from build123d import *

# Parameters (mm, degrees)
SZKIC1_R                        = 23.5
DODANIE_WYCI_GNI_CIE1_DEPTH     = 302
SZKIC2_R                        = 17.5
DODANIE_WYCI_GNI_CIE2_DEPTH     = 50
SZKIC4_R                        = 17.5
DODANIE_WYCI_GNI_CIE3_DEPTH     = 50
SZKIC5_R                        = 5.05
WYTNIJ_WYCI_GNI_CIE1_DEPTH      = 50
SFAZOWANIE1_SIZE                = 2
SZKIC8_R                        = 24
DODANIE_WYCI_GNI_CIE4_DEPTH     = 42.129872
SZKIC12_R                       = 7
DODANIE_WYCI_GNI_CIE5_DEPTH     = 61.69017
SZKIC6_R                        = 11
WYTNIJ_WYCI_GNI_CIE2_DEPTH      = 302
SZKIC13_R                       = 7
DODANIE_WYCI_GNI_CIE6_DEPTH     = 50
DODANIE_WYCI_GNI_CIE7_START     = 14.5
DODANIE_WYCI_GNI_CIE7_DEPTH     = 3
ZAOKR_GLENIE1_R                 = 10
LUSTRO2_START                   = 14.5
LUSTRO2_COPY_1_DEPTH            = 3
WYTNIJ_WYCI_GNI_CIE3_START      = -3
SZKIC17_R                       = 23.5
SZKIC17_R_2                     = 23
WYTNIJ_WYCI_GNI_CIE3_DEPTH      = 8
SZKIC18_R                       = 23.5
SZKIC18_R_2                     = 17
WYTNIJ_WYCI_GNI_CIE4_DEPTH      = 60
WYTNIJ_WYCI_GNI_CIE4_DEPTH_BACK = 95
SZKIC20_R                       = 18.5
WYTNIJ_WYCI_GNI_CIE5_DEPTH      = 45


with BuildPart() as part:
    # Szkic1 → Dodanie-wyciągnięcie1 (new body)
    with BuildSketch(Plane(origin=(0, 0, 0), x_dir=(0, 0, -1), z_dir=(1, 0, 0))):
        Circle(SZKIC1_R)
    extrude(amount=DODANIE_WYCI_GNI_CIE1_DEPTH)

    # Szkic2 → Dodanie-wyciągnięcie2 (add)
    with BuildSketch(Plane.XY):
        with Locations((31, -38)):
            Circle(SZKIC2_R)
    extrude(amount=DODANIE_WYCI_GNI_CIE2_DEPTH)

    # Szkic4 → Dodanie-wyciągnięcie3 (add)
    with BuildSketch(Plane(origin=(0, 0, 0), x_dir=(-1, 0, 0), z_dir=(0, 0, -1))):
        with Locations((-271, -38)):
            Circle(SZKIC4_R)
    extrude(amount=-DODANIE_WYCI_GNI_CIE3_DEPTH)

    # Szkic5 → Wytnij-wyciągnięcie1 (cut)
    with BuildSketch(Plane.XY.offset(50)):
        with Locations((31, -38)):
            Circle(SZKIC5_R)
        with Locations((271, -38)):
            Circle(SZKIC5_R)
    extrude(amount=-WYTNIJ_WYCI_GNI_CIE1_DEPTH, mode=Mode.SUBTRACT)

    # Sfazowanie1
    sfazowanie1_edges = [part.edges().sort_by_distance(p)[0] for p in [
        (25.95, -38, 0),
        (25.95, -38, 50),
        (265.95, -38, 0),
        (265.95, -38, 50),
    ]]
    chamfer(sfazowanie1_edges, length=SFAZOWANIE1_SIZE)

    # Szkic8 → Dodanie-wyciągnięcie4 (add)
    with BuildSketch(Plane(origin=(64.694528313, 23.5, 42), x_dir=(0.996917334, 0, 0.078459096), z_dir=(-0.078459096, 0, 0.996917334))):
        with Locations((0, -13.25)):
            Circle(SZKIC8_R)
    extrude(amount=-DODANIE_WYCI_GNI_CIE4_DEPTH)

    # Szkic12 → Dodanie-wyciągnięcie5 (add)
    with BuildSketch(Plane(origin=(-2.886875267, 0, 36.681228189), x_dir=(0.996917334, 0, 0.078459096), z_dir=(-0.078459096, 0, 0.996917334))):
        with Locations((67.790378694, 10.25)):
            Circle(SZKIC12_R)
    extrude(amount=DODANIE_WYCI_GNI_CIE5_DEPTH)

    # Szkic6 → Wytnij-wyciągnięcie2 (cut)
    with BuildSketch(Plane.ZY):
        Circle(SZKIC6_R)
    extrude(amount=-WYTNIJ_WYCI_GNI_CIE2_DEPTH, mode=Mode.SUBTRACT)

    # Szkic13 → Dodanie-wyciągnięcie6 (add)
    with BuildSketch(Plane(origin=(64.694528313, 23.5, 42), x_dir=(0.996917334, 0, 0.078459096), z_dir=(-0.078459096, 0, 0.996917334))):
        with Locations((0, -13.25)):
            Circle(SZKIC13_R)
    extrude(amount=-DODANIE_WYCI_GNI_CIE6_DEPTH)

    # Szkic16 → Dodanie-wyciągnięcie7 (add)
    with BuildSketch(Plane.ZY.offset(-31).offset(DODANIE_WYCI_GNI_CIE7_START)):
        Polygon((50, -38), (0, -38), (0, -20.172556468), (13.849344331, -17.060101722), (21.580694053, -1.91951259), (17.483252048, 15.703053774), (50, -20.5), align=None)
    dodanie_wyci_gni_cie7 = extrude(amount=DODANIE_WYCI_GNI_CIE7_DEPTH)

    # Zaokrąglenie1
    zaokr_glenie1_edges = [part.edges().sort_by_distance(p)[0] for p in [
        (68.000000001, 34.25, 3.37e-07),
    ]]
    fillet(zaokr_glenie1_edges, radius=ZAOKR_GLENIE1_R)

    # Lustro1: Dodanie-wyciągnięcie7 across plane
    add(dodanie_wyci_gni_cie7.mirror(Plane.ZY.offset(-31)))

    # Lustro2: Dodanie-wyciągnięcie7 across plane
    add(dodanie_wyci_gni_cie7.mirror(Plane.ZY.offset(-151)))

    # Lustro2 copy 1 sketch → Lustro2 copy 1 (add)
    with BuildSketch(Plane.ZY.offset(-271).offset(LUSTRO2_START)):
        Polygon((50, -38), (0, -38), (0, -20.172556468), (13.849344331, -17.060101722), (21.580694053, -1.91951259), (17.483252048, 15.703053774), (50, -20.5), align=None)
    extrude(amount=LUSTRO2_COPY_1_DEPTH)

    # Szkic17 → Wytnij-wyciągnięcie3 (cut)
    with BuildSketch(Plane.ZY.offset(WYTNIJ_WYCI_GNI_CIE3_START)):
        Circle(SZKIC17_R)
        Circle(SZKIC17_R_2, mode=Mode.SUBTRACT)
    wytnij_wyci_gni_cie3 = extrude(amount=-WYTNIJ_WYCI_GNI_CIE3_DEPTH, mode=Mode.SUBTRACT)

    # Lustro3: Wytnij-wyciągnięcie3 across plane
    add(wytnij_wyci_gni_cie3.mirror(Plane.ZY.offset(-151)), mode=Mode.SUBTRACT)

    # Szkic18 → Wytnij-wyciągnięcie4 (cut, two sides)
    with BuildSketch(Plane.ZY.offset(-151)) as wytnij_wyci_gni_cie4_sk:
        Circle(SZKIC18_R)
        Circle(SZKIC18_R_2, mode=Mode.SUBTRACT)
    extrude(amount=WYTNIJ_WYCI_GNI_CIE4_DEPTH, mode=Mode.SUBTRACT)
    extrude(wytnij_wyci_gni_cie4_sk.sketch, amount=-WYTNIJ_WYCI_GNI_CIE4_DEPTH_BACK, mode=Mode.SUBTRACT)

    # Szkic19 → Obrót1 (revolve)
    with BuildSketch(Plane.XY):
        Polygon((91, 23.5), (91, 17), (121, 17), align=None)
        Polygon((246, 17), (246, 23.5), (236, 17), align=None)
    revolve(axis=Axis((0, 0, 0), (1, 0, 0)))

    # Szkic20 → Wytnij-wyciągnięcie5 (cut)
    with BuildSketch(Plane.ZY):
        Circle(SZKIC20_R)
    wytnij_wyci_gni_cie5 = extrude(amount=-WYTNIJ_WYCI_GNI_CIE5_DEPTH, mode=Mode.SUBTRACT)

    # Lustro4: Wytnij-wyciągnięcie5 across plane
    add(wytnij_wyci_gni_cie5.mirror(Plane.ZY.offset(-151)), mode=Mode.SUBTRACT)


solid = part.part
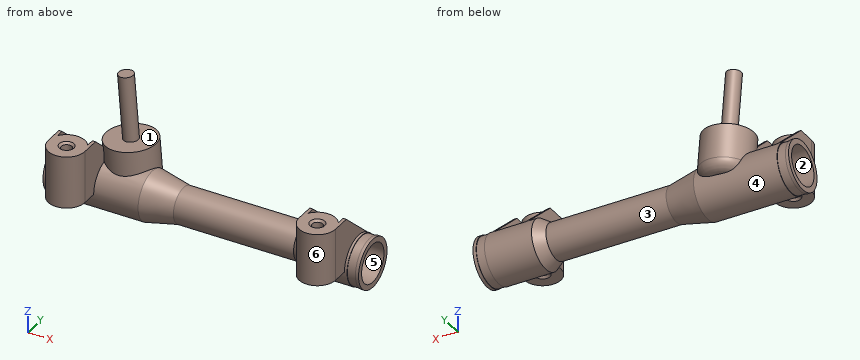
Check sheet for the modelled part. Datum: model origin and axes. Units: mm. Face numbers are marked on the shaded views. A direction names the side the tool comes from. Give positions to 0.01 mm unless a question says otherwise; leave off trailing zeros. Order: outer loops, then holes, each group sorted by start corner. A loop starts at its lowest first (then second) coordinate and runs counter-clockwise, first axis right, second up. Notation, with made-up numbers: (30.5, 45.25) - (43.5, 45.25) arc R9 ccw to (43.5, 51.25) - close; hole circle Ø5 at (47.5, -24). An arc over 180 degrees is marked (long way). Answer as CSV lines item,"result".
1. Mould release check, pull along Y, two halves, no side actions. Record for the marked faces 1, 2 and 3: released by +Y, released by -Y, zero draft, split by the parting line, or undercut.
Result sheet:
face 1,"zero draft"
face 2,"undercut"
face 3,"split by the parting line"
2. Tool access check on the marked faces 4, 5 and 6. Record the directions out of +Z, -Z, +X, -X, +Y, -Y that give a thin tool (end or side, any length) a straight path to the whole face; none if there is none.
Result sheet:
face 4,"none"
face 5,"+X"
face 6,"+Z, -Z, -Y"
3. Go/stop test with flat-tipped pins: P1, Ø5, axis at y = 8.5, z = 11, coming from the +X side; P2, Ø11.5, axis at x = 31, y = -38, coming from the -Z side; P3, Ø15, axis at y = -7, z = 34.5, coming from the +X side; P4, Ø12, axis at x = 243.5, y = -33, coming from the -Z side. Record where each tip stops, or that it passes through.
Result sheet:
P1,"x = 257"
P2,"z = 1.3"
P3,"x = 288.5"
P4,"through"
4. Section check A-A (x = 31). Record the boundary of the cut face in (y, z).
Result sheet:
outline,"(-55.5, 0) - (-45.05, 0) - (-43.05, 2) - (-43.05, 48) - (-45.05, 50) - (-55.5, 50) - close; (-32.95, 2) - (-30.95, 0) - (-23.5, 0) arc R23.5 ccw (long way) to (-20.5, 11.49) - (-20.5, 50) - (-30.95, 50) - (-32.95, 48) - close; hole circle Ø37 at (0, 0)"
5. Section check B-B (y = -49). Record the boundary of the cut face in (x, z).
Result sheet:
outline,"(17.39, 0) - (44.61, 0) - (44.61, 50) - (17.39, 50) - close; (257.39, 0) - (284.61, 0) - (284.61, 50) - (257.39, 50) - close"
6. Section check C-C (x = 162.5). Record the boundary of the cut face in (y, z).
Result sheet:
outline,"circle Ø34 at (0, 0); hole circle Ø22 at (0, 0)"
7. Scan lines: probe 1 along Y at (x, z) = (31, 36.5); probe 2 along Z at (x, y) = (179, -1); probe 3 along Z at (x, y) = (239, -2). Record each from-to range of solid material in increasing order. Write a range as from..to.
Result sheet:
probe 1,"-55.5..-43.05, -32.95..-20.5"
probe 2,"-16.97..-10.95, 10.95..16.97"
probe 3,"-18.84..-10.82, 10.82..18.84"
